Could you check a few things on this model? Use its own coordinates, in mm. A direction names the side the tool comes from. Give positions to 0.01 mm unless a question says otherwise; leave off trailing zeros. Order: outer loops, then holes, each group sorted by start corner. A loop starts at its lowest first (then second) coordinate and runs counter-clockwise, first axis right, second up. Notation, with made-up numbers: M 73.5,45.25 L 119.5,45.25 A7 ccw 119.5,51.25 Z; hole C -40,78 d3. An arc over 180 degrees is marked long. Return JSON: item names as keys, results as strings. Group by question number.
Autodesk Inventor part; units mm, degrees
ref_plane "YZ Plane" through (0, 0, 0) normal (1, 0, 0) x (0, 1, 0)
ref_plane "XZ Plane" through (0, 0, 0) normal (0, 1, 0) x (-1, 0, 0)
ref_plane "XY Plane" through (0, 0, 0) normal (0, 0, 1) x (1, 0, 0)
sketch "Esboço1" plane through (0, 0, 0) normal (0, 0, 1) x (1, 0, 0)
  line L0 (-55, 14.75) -> (52, 14.75)
  line L1 (52, 14.75) -> (52, -18)
  line L2 (52, -18) -> (-55, -18)
  line L3 (-55, -18) -> (-55, 14.75)
  line L4 (52.0001, 13.75) -> (52.0001, 10.75)
  line L5 (-50.5, -18) -> (-53.5, -18)
  point P0 (0, 0)
  dimension "d34" = 52
  dimension "d35" = 18
  dimension "d36" = 14.75
extrude "Extrusão1" add sketch "Esboço1" along normal blind 3
sketch "Esboço2" plane through (0, 0, 3) normal (0, 0, 1) x (1, 0, 0)
  line L0 (19.2209, 13.75) -> (19.2209, 10.75)
  line L1 (52, 14.75) -> (-55, 14.75)
  line L2 (-55, 14.75) -> (-55, -18)
  line L3 (-55, 14.75) -> (-43.2, 14.75)
  line L4 (-43.2, 14.75) -> (-43.2, 10.75)
  line L5 (-43.2, 10.75) -> (-55, 10.75)
  line L6 (-55, 10.75) -> (-55, 14.75)
  line L7 (-19.4, 14.75) -> (-19.4, 10.75)
  line L8 (-19.4, 10.75) -> (-31.2, 10.75)
  line L9 (-31.2, 10.75) -> (-31.2, 14.75)
  line L10 (-31.2, 14.75) -> (-19.4, 14.75)
  line L11 (4.4, 14.75) -> (4.4, 10.75)
  line L12 (4.4, 10.75) -> (-7.4, 10.75)
  line L13 (-7.4, 10.75) -> (-7.4, 14.75)
  line L14 (-7.4, 14.75) -> (4.4, 14.75)
  line L15 (28.2, 14.75) -> (28.2, 10.75)
  line L16 (28.2, 10.75) -> (16.4, 10.75)
  line L17 (16.4, 10.75) -> (16.4, 14.75)
  line L18 (16.4, 14.75) -> (28.2, 14.75)
  line L19 (-55, -18) -> (-43.2, -18)
  line L20 (-43.2, -18) -> (-43.2, -14.869)
  line L21 (-43.2, -14.869) -> (-55, -14.869)
  line L22 (-55, -14.869) -> (-55, -18)
  line L23 (-19.4, -18) -> (-19.4, -14.869)
  line L24 (-31.2, -18) -> (-19.4, -18)
  line L25 (-31.2, -14.869) -> (-31.2, -18)
  line L26 (-19.4, -14.869) -> (-31.2, -14.869)
  line L27 (4.4, -18) -> (4.4, -14.869)
  line L28 (-7.4, -18) -> (4.4, -18)
  line L29 (-7.4, -14.869) -> (-7.4, -18)
  line L30 (4.4, -14.869) -> (-7.4, -14.869)
  line L31 (28.2, -18) -> (28.2, -14.869)
  line L32 (16.4, -18) -> (28.2, -18)
  line L33 (16.4, -14.869) -> (16.4, -18)
  line L34 (28.2, -14.869) -> (16.4, -14.869)
  line L35 (52, -18) -> (52, -14.869)
  line L36 (40.2, -18) -> (52, -18)
  line L37 (40.2, -14.869) -> (40.2, -18)
  line L38 (52, -14.869) -> (40.2, -14.869)
  line L39 (-53.4999, 2.375) -> (-50.4999, 2.375)
  line L40 (-50.4999, 2.375) -> (-50.4999, -9.625)
  line L41 (-50.4999, -9.625) -> (-53.4999, -9.625)
  line L42 (-53.4999, 2.375) -> (-53.4999, -9.625)
  line L43 (-53.4999, -9.625) -> (-50.4999, -9.625)
  line L44 (-50.4999, -9.625) -> (-50.4999, 2.375)
  line L45 (-50.4999, 2.375) -> (-53.4999, 2.375)
  line L46 (-53.4999, 2.375) -> (-53.4999, -9.625)
  line L47 (52, 14.75) -> (52, 10.75)
  line L48 (52, 10.75) -> (40.2, 10.75)
  line L49 (40.2, 10.75) -> (40.2, 14.75)
  line L50 (40.2, 14.75) -> (52, 14.75)
  line L51 (51, 5.506) -> (48, 5.506)
  line L52 (48, 5.506) -> (48, -6.494)
  line L53 (48, -6.494) -> (51, -6.494)
  line L54 (51, 5.506) -> (51, -6.494)
  line L55 (48, 5.506) -> (51, 5.506)
  line L56 (51, 5.506) -> (51, -6.494)
  line L57 (51, -6.494) -> (48, -6.494)
  line L58 (48, -6.494) -> (48, 5.506)
  point P0 (52, -18)
  point P1 (4.4, 14.75)
  point P2 (-43.2, 14.75)
  dimension "d37" = 11.8
  dimension "d38" = 4
  dimension "d41" = 23.8
  dimension "d46" = 11.8
  dimension "d49" = 23.8
extrude "Extrusão2" cut sketch "Esboço2" against normal through all
properties part number "Acrilico-Parachoque-Parede-Inf"
1. Imagine slicing it at B-B, the plane y = -5. Please give me the cut outline in (x, z), plus the area to 3 significant figures.
2. Imagine slicing it at A-A, the plane y = 12. Please give me the cut outline in (x, z).
3. For pin 1 (1.5 mm diameter, centred on y = 13, z = 1.5, fed in from -X); pin 2 (1.5 mm diameter, centred on x = -0.5, z = 2, fed in from -Y); pin 3 (1.5 mm diameter, centred on y = -16, z = 1.5, fed in from +X), each with a flat end and sliding along its axis, tell me the tip position at first contact or that it passes through.
4. Imagine slicing it at D-D, the plane x = -27. Please give me the cut outline in (y, z).
5. If we mould it in two halves opening along X, with no side actions, what happens to faces 5 (the flat face through (40.2, -16, 2)), 6 (the flat face through (34, -18, 1)), 7 (the flat face through (28.2, 13, 2))? For each: pulls with the +X half, pulls with the -X half, needs draft (parallel to the pull), parting line crosses it, or undercut.
6. Which directions (+Z, -Z, +X, -X, +Y, -Y) give clear straight access to the entire face, cutting with the end or side of a thin tool? Please do faces 1 (the flat face through (51, 0, 2)), 2 (the flat face through (22, -14.869, 2)), 3 (the flat face through (46, -14.869, 2)), 4 (the flat face through (-1, 10.75, 2)).
7. Imagine slicing it at C-C, the plane z = 2.2. Count the separate pieces of the cut face and the enclosed holes in it, plus the area to 3 significant figures.
8. I need wall thicknesses on L1, parallel to X at y = 2, z = 2.35; L2, parallel to X at y = 12, z = 0.7; L3, parallel to X at y = -8, z = 1. Which ranges of each line are inside material? Lowest first, please. Write a range as from..to.
Values:
{
 "1": {"outline": "M -55,0 L -53.5,0 L -53.5,3 L -55,3 Z; M -50.5,0 L 48,0 L 48,3 L -50.5,3 Z; M 51,0 L 52,0 L 52,3 L 51,3 Z", "area": "303 mm²"},
 "2": {"outline": "M -43.2,0 L -31.2,0 L -31.2,3 L -43.2,3 Z; M -19.4,0 L -7.4,0 L -7.4,3 L -19.4,3 Z; M 4.4,0 L 16.4,0 L 16.4,3 L 4.4,3 Z; M 28.2,0 L 40.2,0 L 40.2,3 L 28.2,3 Z"},
 "3": {"pin 1": "stops at x = -43.2", "pin 2": "stops at y = -14.87", "pin 3": "stops at x = 40.2"},
 "4": {"outline": "M -14.87,0 L 10.75,0 L 10.75,3 L -14.87,3 Z"},
 "5": {"face 5": "pulls with the +X half", "face 6": "needs draft", "face 7": "undercut"},
 "6": {"face 1": "+Z, -Z", "face 2": "+Z, -Z, -Y", "face 3": "+Z, -Z, +X, -Y", "face 4": "+Z, -Z, +Y"},
 "7": {"separate pieces": "1", "enclosed holes": "2", "area": "3,010 mm²"},
 "8": {"L1": "x = -55..-53.5, -50.5..48, 51..52", "L2": "x = -43.2..-31.2, -19.4..-7.4, 4.4..16.4, 28.2..40.2", "L3": "x = -55..-53.5, -50.5..52"}
}
